```python
from build123d import *

# Parameters (mm, degrees)
F0_R     = 63.5
F1_DEPTH = 1.905
F2_R     = 2.38125
F3_DEPTH = 1.906
F4_R     = 63.5
F4_R_2   = 60.96
F5_DEPTH = 2.54


# Not quite as in the source:
# - a fillet or chamfer that OpenCascade refuses, or shapes differently, is made with other operations: its cross-section is extruded or revolved along the edge and cut away or added


with BuildPart() as f1:
    # F0 (on Top) → F1 (new body)
    with BuildSketch(Plane.XY):
        Circle(F0_R)
    extrude(amount=F1_DEPTH)

    # F2 (on face) → F3 (cut, through all)
    with BuildSketch(Plane.XY.offset(1.905)):
        with Locations((0, 44.45)):
            Circle(F2_R)
        with Locations((0, -44.45)):
            Circle(F2_R)
    extrude(amount=-F3_DEPTH, mode=Mode.SUBTRACT)

    # F4 (on face) → F5 (join)
    with BuildSketch(Plane(origin=(0, 0, 0), x_dir=(1, 0, 0), z_dir=(0, 0, -1))):
        Circle(F4_R)
        Circle(F4_R_2, mode=Mode.SUBTRACT)
    extrude(amount=F5_DEPTH)

    # F6: fillet of radius 5.08 on 1 edges, made by hand

    # F6_s1 → F6_t2 (revolve, cut)
    with BuildSketch(Plane.XZ):
        with BuildLine():
            ThreePointArc((63.5, -2.54), (61.8199479175, 0.635), (58.4598437524, 1.905))
            Line((58.4598437524, 1.905), (63.5, 1.905))
            Line((63.5, 1.905), (63.5, -2.54))
        make_face()
    revolve(axis=Axis((0, 0, 1.905), (0, 0, 1)), mode=Mode.SUBTRACT)


solid = f1.part
```
Read the model definition and answer for the solid it produces. Units are mm, in the model's axes. A direction names the side the tool comes from. Give positions to 0.01 mm unless a question says otherwise; leave off trailing zeros. Loops run counter-clockwise (first coordinate to the right, second up) from the corner with the lowest first, then second, coordinate; pieces in that order, holes last.
Item 1: The part is cut by section C-C (z = -0.7). Write down the section's boundary in (x, y).
Item 2: Each of these flat-tipped pins is pushed along its axis until it touches: pin 1 Ø1 at (y, z) = (35.5, 0.5) entering from +X; pin 2 Ø2 at (x, z) = (-1.5, -0.5) entering from +Y; pin 3 Ø2 at (y, z) = (40, 1) entering from +X. Where does it stop, or does it pass through?
Item 3: For faces 3 (the flat face through (-1, 1, 0)), 4 (the cylindrical face through (-0.516, 42.125, 0.966)), determine the directions among +Z, -Z, +X, -X, +Y, -Y from which every point of the face is accessible in a straight line to the end or side of a thin tool.
Item 4: The mould has two halves that part along X. Classify faces 1 (the flat face through (-24, -57, -2.54)), 2 (the cylindrical face through (-0.31, -42.09, 0.97)): released by +X, released by -X, zero draft, split by the parting line, or undercut.
Item 5: The part is cut by section B-B (y = 0). Write down the section's boundary in (x, z) (3 decimals).
Item 6: Find the intervals of material crossed by line 1 along Y through (x, z) = (0, 0.65); line 2 along Y through (x, z) = (0, 0.85); line 3 along Z through (x, y) = (-35, -32.5) (3 decimals), in increasing order.
Item 7: The part is cut by section A-A (x = 0). Write down the section's boundary in (y, z) (3 decimals), and give its area (3 significant figures).
Taken from the geometry:
1. outline: circle Ø125.79 at (0, 0); hole circle Ø121.92 at (0, 0)
2. pin 1: stops at x = 51.46
2. pin 2: stops at y = 63.24
2. pin 3: stops at x = 48.2
3. face 3: -Z
3. face 4: +Z, -Z
4. face 1: zero draft
4. face 2: undercut
5. outline: (-63.5, -2.54) - (-60.96, -2.54) - (-60.96, 0) - (60.96, 0) - (60.96, -2.54) - (63.5, -2.54) arc R5.08 ccw to (58.46, 1.905) - (-58.46, 1.905) arc R5.08 ccw to start
6. line 1: y = -61.8 to -46.83, -42.07 to 42.07, 46.83 to 61.8
6. line 2: y = -61.56 to -46.83, -42.07 to 42.07, 46.83 to 61.56
6. line 3: z = 0 to 1.905
7. outline: (-63.5, -2.54) - (-60.96, -2.54) - (-60.96, 0) - (-46.831, 0) - (-46.831, 1.905) - (-58.46, 1.905) arc R5.08 ccw to start; (-42.069, 0) - (42.069, 0) - (42.069, 1.905) - (-42.069, 1.905) - close; (46.831, 0) - (60.96, 0) - (60.96, -2.54) - (63.5, -2.54) arc R5.08 ccw to (58.46, 1.905) - (46.831, 1.905) - close
7. area: 226 mm2
